The model under review builds one solid part; all positions refer to its coordinate system, in mm. Face numbers are marked on the shaded views. A direction names the side the tool comes from. Give positions to 0.01 mm unless a question says otherwise; leave off trailing zeros. Loops run counter-clockwise (first coordinate to the right, second up) from the corner with the lowest first, then second, coordinate; pieces in that order, holes last. Notation, with made-up numbers: M -39.5,-34.75 L -0.5,-34.75 A22 cw -0.5,-11.75 Z; hole C 67.25,-34.75 d1. An arc over 180 degrees is marked long. Return JSON: item names as keys, results as strings. Group by question number.
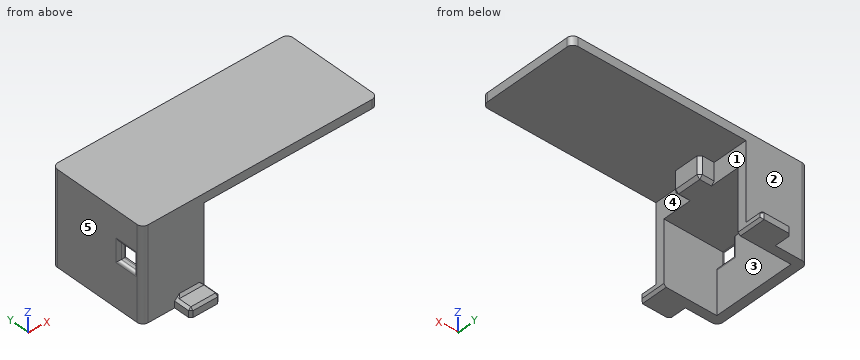
```python
from build123d import *

# Parameters (mm, degrees)
BOSS_EXTRUDE1_DEPTH      = 21.59
BOSS_EXTRUDE1_DEPTH_BACK = 21.59
BOSS_EXTRUDE2_DEPTH      = 6.35
BOSS_EXTRUDE2_DEPTH_BACK = 6.35
SKETCH1_4_W              = 6.35
SKETCH1_4_H              = 3.81
SKETCH3_W                = 26.67
SKETCH3_H                = 31.242
BOSS_EXTRUDE3_DEPTH      = 3.81
FILLET1_R                = 2.54
CHAMFER1_SIZE            = 1.27
SKETCH9_W                = 12.7
SKETCH9_H                = 3.81
BOSS_EXTRUDE6_DEPTH      = 7.62
CHAMFER2_SIZE            = 1.016
CHAMFER3_SIZE            = 1.016
CHAMFER2_OF_MIRROR2_SIZE = 1.016
BOSS_EXTRUDE7_START      = 5.08
BOSS_EXTRUDE7_DEPTH      = 5.08
BOSS_EXTRUDE8_START      = 3.81
BOSS_EXTRUDE8_DEPTH      = 3.81
CHAMFER4_SIZE            = 1.016
SKETCH12_W               = 7.62
SKETCH12_H               = 7.62
CUT_EXTRUDE2_DEPTH       = 3.81
FILLET8_R                = 1.27


with BuildPart() as part:
    # Sketch1 → Boss-Extrude1 (new, two sides: drawn at the far end of the back side and taken through both)
    with BuildSketch(Plane(origin=(0, 0, 0), x_dir=(1, 0, 0), z_dir=(0, 1, 0)).offset(-BOSS_EXTRUDE1_DEPTH_BACK)):
        Polygon((-16.51, 31.242), (-16.51, 0), (10.16, 0), (10.16, 3.81), (-12.7, 3.81), (-12.7, 31.242), align=None)
    extrude(amount=BOSS_EXTRUDE1_DEPTH + BOSS_EXTRUDE1_DEPTH_BACK)

    # Sketch1<4> → Boss-Extrude2 (add, two sides: drawn at the far end of the back side and taken through both)
    with BuildSketch(Plane(origin=(0, 0, 0), x_dir=(1, 0, 0), z_dir=(0, 1, 0)).offset(-BOSS_EXTRUDE2_DEPTH_BACK)):
        with Locations((13.335, 1.905)):
            Rectangle(SKETCH1_4_W, SKETCH1_4_H)
    extrude(amount=BOSS_EXTRUDE2_DEPTH + BOSS_EXTRUDE2_DEPTH_BACK)

    # Sketch3 → Boss-Extrude3 (add)
    with BuildSketch(Plane(origin=(0, 21.59, 0), x_dir=(1, 0, 0), z_dir=(0, 1, 0))):
        with Locations((-3.175, 15.621)):
            Rectangle(SKETCH3_W, SKETCH3_H)
    boss_extrude3 = extrude(amount=-BOSS_EXTRUDE3_DEPTH)

    # Mirror1: Boss-Extrude3 across plane
    add(boss_extrude3.mirror(Plane.ZX))

    # Fillet1
    fillet1_edges = [part.edges().sort_by_distance(p)[0] for p in [
        (-16.51, -21.59, -15.621),
        (-16.51, 21.59, -15.621),
    ]]
    fillet(fillet1_edges, radius=FILLET1_R)

    # Chamfer1
    chamfer1_edges = [part.edges().sort_by_distance(p)[0] for p in [
        (13.335, -6.35, -3.81),
        (16.51, 0, -3.81),
        (16.51, -6.35, -1.905),
        (13.335, 6.35, -3.81),
        (16.51, 6.35, -1.905),
    ]]
    chamfer(chamfer1_edges, length=CHAMFER1_SIZE)

    # Sketch9 → Boss-Extrude6 (add)
    with BuildSketch(Plane.XZ.offset(21.59)):
        with Locations((3.81, -29.337)):
            Rectangle(SKETCH9_W, SKETCH9_H)
    boss_extrude6 = extrude(amount=BOSS_EXTRUDE6_DEPTH)

    # Chamfer2
    chamfer2_edges = [part.edges().sort_by_distance(p)[0] for p in [
        (10.16, -25.4, -27.432),
        (-2.54, -25.4, -27.432),
        (10.16, -29.21, -29.337),
        (3.81, -29.21, -27.432),
        (-2.54, -29.21, -29.337),
    ]]
    chamfer(chamfer2_edges, length=CHAMFER2_SIZE)

    # Chamfer3
    chamfer3_edges = [part.edges().sort_by_distance(p)[0] for p in [
        (3.81, -21.59, -27.432),
        (10.16, -22.987, -31.242),
    ]]
    chamfer(chamfer3_edges, length=CHAMFER3_SIZE)

    # Mirror2: Boss-Extrude6 across plane
    add(boss_extrude6.mirror(Plane.ZX))

    # Chamfer2 of Mirror2
    chamfer2_of_mirror2_edges = [part.edges().sort_by_distance(p)[0] for p in [
        (10.16, 25.4, -27.432),
        (-2.54, 25.4, -27.432),
        (10.16, 29.21, -29.337),
        (3.81, 29.21, -27.432),
        (-2.54, 29.21, -29.337),
    ]]
    chamfer(chamfer2_of_mirror2_edges, length=CHAMFER2_OF_MIRROR2_SIZE)

    # Sketch10 → Boss-Extrude7 (add)
    with BuildSketch(Plane.XY.offset(BOSS_EXTRUDE7_START)):
        with BuildLine():
            Line((10.16, 6.35), (10.16, 21.59))
            Line((10.16, 21.59), (-13.97, 21.59))
            ThreePointArc((-13.97, 21.59), (-15.766051224, 20.846051224), (-16.51, 19.05))
            Line((-16.51, 19.05), (-16.51, -19.05))
            ThreePointArc((-16.51, -19.05), (-15.766051224, -20.846051224), (-13.97, -21.59))
            Line((-13.97, -21.59), (10.16, -21.59))
            Line((10.16, -21.59), (10.16, -6.35))
            Line((10.16, -6.35), (15.24, -6.35))
            Line((15.24, -6.35), (16.51, -5.08))
            Line((16.51, -5.08), (16.51, 5.08))
            Line((16.51, 5.08), (15.24, 6.35))
            Line((15.24, 6.35), (10.16, 6.35))
        make_face()
    extrude(amount=-BOSS_EXTRUDE7_DEPTH)

    # Sketch11 → Boss-Extrude8 (add)
    with BuildSketch(Plane.XY.offset(5.08).offset(BOSS_EXTRUDE8_START)):
        with BuildLine():
            Line((-13.97, 21.59), (82.55, 21.59))
            ThreePointArc((82.55, 21.59), (84.346051224, 20.846051224), (85.09, 19.05))
            Line((85.09, 19.05), (85.09, -19.05))
            ThreePointArc((85.09, -19.05), (84.346051224, -20.846051224), (82.55, -21.59))
            Line((82.55, -21.59), (-13.97, -21.59))
            ThreePointArc((-13.97, -21.59), (-15.766051224, -20.846051224), (-16.51, -19.05))
            Line((-16.51, -19.05), (-16.51, 19.05))
            ThreePointArc((-16.51, 19.05), (-15.766051224, 20.846051224), (-13.97, 21.59))
        make_face()
    extrude(amount=-BOSS_EXTRUDE8_DEPTH)

    # Chamfer4
    chamfer4_edges = [part.edges().sort_by_distance(p)[0] for p in [
        (3.81, 21.59, -27.432),
        (10.16, 22.987, -31.242),
    ]]
    chamfer(chamfer4_edges, length=CHAMFER4_SIZE)

    # Sketch12 → Cut-Extrude2 (cut)
    with BuildSketch(Plane(origin=(-12.7, 0, 0), x_dir=(0, 0, -1), z_dir=(1, 0, 0))):
        with Locations((7.62, -13.97)):
            Rectangle(SKETCH12_W, SKETCH12_H)
    extrude(amount=-CUT_EXTRUDE2_DEPTH, mode=Mode.SUBTRACT)

    # Fillet8
    fillet8_edges = [part.edges().sort_by_distance(p)[0] for p in [
        (-12.7, -13.97, -11.43),
        (-12.7, -10.16, -7.62),
        (-16.51, -17.78, -7.62),
        (-16.51, -13.97, -11.43),
        (-16.51, -10.16, -7.62),
        (-16.51, -13.97, -3.81),
    ]]
    fillet(fillet8_edges, radius=FILLET8_R - 0.0001)  # a hair under: the kernel refuses the full size


solid = part.part
```
(1) For pin 1 (1.5 mm diameter, centred on x = 52.5, y = -5, fed in from -Z); pin 2 (0.8 mm diameter, centred on y = -26, z = -30, fed in from -X); pin 3 (5.5 mm diameter, centred on x = 13, z = 1.5, fed in from +Y), all flat-tipped, find the tip position at first contact; note any pin that passes through.
(2) Add section D-D (z = -22.5). Write out the cut boundary in (x, y).
(3) Add section A-A (y = -14.5). Write out the cut boundary in (x, z).
(4) Add section C-C (y = 12). Write out the cut boundary in (x, z).
(5) For the marked faces 4 and 5, list the 3-axis set-ups (+Z, -Z, +X, -X, +Y, -Y) from which the entire face can be reached by the end or side of a thin tool; tool diameter is ignored.
(6) Mouldability with a two-part tool opening along Y and no side actions: class the marked faces 1, 2 and 3 as released by +Y, released by -Y, zero draft, split by the parting line, or undercut.
(7) For probe 1 along X at (y, z) = (3, 2.5); probe 2 along Y at (x, z) = (63, 6); probe 3 along Y at (x, z) = (4.5, -4), list the stretches that pass through material, from the lowest coordinate up.
Verdict:
{
 "1": {"pin 1": "stops at z = 5.08", "pin 2": "stops at x = -2.54", "pin 3": "stops at y = 6.35"},
 "2": {"outline": "M -16.51,-19.05 A2.54 ccw -13.97,-21.59 L 10.16,-21.59 L 10.16,-17.78 L -12.7,-17.78 L -12.7,17.78 L 10.16,17.78 L 10.16,21.59 L -13.97,21.59 A2.54 ccw -16.51,19.05 Z"},
 "3": {"outline": "M -16.51,-31.24 L -12.7,-31.24 L -12.7,-12.7 A1.27 ccw -13.97,-11.43 L -15.24,-11.43 A1.27 ccw -16.51,-12.7 Z; M -16.51,-2.54 A1.27 ccw -15.24,-3.81 L 10.16,-3.81 L 10.16,5.08 L 85.09,5.08 L 85.09,8.89 L -16.51,8.89 Z"},
 "4": {"outline": "M -16.51,-31.24 L -12.7,-31.24 L -12.7,-3.81 L 10.16,-3.81 L 10.16,5.08 L 85.09,5.08 L 85.09,8.89 L -16.51,8.89 Z"},
 "5": {"face 4": "-Z, +X, -Y", "face 5": "+Z, -Z, -X, +Y, -Y"},
 "6": {"face 1": "zero draft", "face 2": "released by +Y", "face 3": "undercut"},
 "7": {"probe 1": "x = -16.51 to 16.51", "probe 2": "y = -21.59 to 21.59", "probe 3": "y = -21.59 to -17.78, 17.78 to 21.59"}
}
